For this review, take the finished solid that the model builds, in its own axes (mm). A direction names the side the tool comes from. Round coordinates to 2 decimals unless told otherwise and drop trailing zeros. Loops run counter-clockwise (first coordinate to the right, second up) from the corner with the lowest first, then second, coordinate; pieces in that order, holes last.
```python
from build123d import *

# Parameters (mm, degrees)
SKETCH_1_W          = 2390
SKETCH_1_H          = 1030
EXTRUDE_1_DEPTH     = 950
SKETCH_2_W          = 1790
SKETCH_2_H          = 780
CUT_EXTRUDE_1_DEPTH = 616
SKETCH_3_W          = 300
SKETCH_3_H          = 780
CUT_EXTRUDE_2_DEPTH = 464


with BuildPart() as part:
    # Эскиз1 → Бобышка-Вытянуть1 (new body)
    with BuildSketch(Plane(origin=(0, 0, 0), x_dir=(1, 0, 0), z_dir=(0, 1, 0))):
        with Locations((1195, 515)):
            Rectangle(SKETCH_1_W, SKETCH_1_H)
    extrude(amount=EXTRUDE_1_DEPTH)

    # Эскиз2 → Вырез-Вытянуть1 (cut)
    with BuildSketch(Plane(origin=(0, 950, 0), x_dir=(1, 0, 0), z_dir=(0, 1, 0))):
        with Locations((1195, 390)):
            Rectangle(SKETCH_2_W, SKETCH_2_H)
    extrude(amount=-CUT_EXTRUDE_1_DEPTH, mode=Mode.SUBTRACT)

    # Эскиз3 → Вырез-Вытянуть2 (cut)
    with BuildSketch(Plane(origin=(0, 950, 0), x_dir=(1, 0, 0), z_dir=(0, 1, 0))):
        with Locations((150, 390)):
            Rectangle(SKETCH_3_W, SKETCH_3_H)
        with Locations((2240, 390)):
            Rectangle(SKETCH_3_W, SKETCH_3_H)
    extrude(amount=-CUT_EXTRUDE_2_DEPTH, mode=Mode.SUBTRACT)


solid = part.part
```
(1) The part is to be moulded in two halves that separate along X. For faces 4 (the flat face through (1178, 646, -780)), 5 (the flat face through (300, 411, -385)), 6 (the flat face through (1178, 0, -522)), 7 (the flat face through (0, 363, -622)), say which applies: pulls with the +X half, pulls with the -X half, needs draft (parallel to the pull), parting line crosses it, or undercut.
(2) Add section D-D (x = 2161). Give the boundary of the cut face in (y, z).
(3) Add section C-C (y = 604.5). Give the boundary of the cut face in (x, z), plus the area to 4 significant figures.
(4) For faces 1 (the flat face through (2390, 363, -622)), 2 (the flat face through (148, 486, -395)), 3 (the flat face through (1182, 334, -395)), list the 3-axis set-ups (+Z, -Z, +X, -X, +Y, -Y) from which the entire face can be reached by the end or side of a thin tool; tool diameter is ignored.
(5) Add section A-A (x = 1348). Give the boundary of the cut face in (y, z).
(6) Insertion check: pin 1 Ø8 at (x, z) = (1298.5, -255) entering from +Y; pin 2 Ø2 at (x, z) = (266, -156) entering from +Y; pin 3 Ø10 at (x, y) = (1345.5, 644.5) entering from +Z. Each pin has a flat end and moves straight along its axis. Give the tip position at first contact, or say it passes through.
(7) Add section B-B (z = -241.5). Give the boundary of the cut face in (x, y), plus the area to 3 significant figures.
(8) For L1, parallel to X at y = 383.5, z = -494; L2, parallel to Z at x = 1684, y = 659; L3, parallel to Y at x = 1826, z = -173.5, list the stretches that pass through material, from the lowest coordinate up.
Outcome:
1. face 4: undercut
1. face 5: undercut
1. face 6: needs draft
1. face 7: pulls with the -X half
2. outline: (0, -1030) - (950, -1030) - (950, -780) - (486, -780) - (486, 0) - (0, 0) - close
3. outline: (0, -1030) - (2390, -1030) - (2390, -780) - (0, -780) - close
3. area: 597,500 mm2
4. face 1: +Z, -Z, +X, +Y, -Y
4. face 2: +Z, +X, -X, +Y
4. face 3: +Z, +Y
5. outline: (0, -1030) - (950, -1030) - (950, -780) - (334, -780) - (334, 0) - (0, 0) - close
6. pin 1: stops at y = 334
6. pin 2: stops at y = 486
6. pin 3: stops at z = -780
7. outline: (0, 0) - (2390, 0) - (2390, 486) - (2090, 486) - (2090, 334) - (300, 334) - (300, 486) - (0, 486) - close
7. area: 889,000 mm2
8. L1: x = 0 to 300, 2090 to 2390
8. L2: z = -1030 to -780
8. L3: y = 0 to 334
